Read the model definition and answer for the solid it produces. Units are mm, in the model's axes. A direction names the side the tool comes from. Coordinates: 2 decimals unless noted, no trailing zeros. Write each loop counter-clockwise with the first axis right and the second up, starting at its lowest first coordinate (ties: lowest second). Pieces come first, ordered by that corner, then holes.
(1) Given pin 1 (5.5 mm diameter, centred on y = 16.5, z = -23.5, fed in from +X); pin 2 (6 mm diameter, centred on x = 5.5, z = -14, fed in from +Y); pin 3 (2 mm diameter, centred on x = 3, y = 2.5, fed in from -Z); pin 4 (3.5 mm diameter, centred on x = -1.5, z = -19.5, fed in from -Y), each flat-ended and moving along its own axis, determine where each tip first touches the part or whether it passes through.
(2) Determine the mould class of faces 6 (the cylindrical face through (15.08, 0.09, -4.19)), 7 (the flat face through (-2, 20, -36.5)), 8 (the cylindrical face through (-1.522, 19.546, -32.085)) for opening direction Z: pulls with the +Z half, pulls with the -Z half, needs draft (parallel to the pull), parting line crosses it, or undercut.
(3) The part is cut by section B-B, the plane y = 0. Determine the outline of the cut face in (x, z), and give its area (3 significant figures).
(4) Which of the six approach directions +Z, -Z, +X, -X, +Y, -Y give full straight-line access (tool end or side, diameter ignored) to faces 1 (the flat face through (-10, 4.25, -4)), 2 (the flat face through (-1, 6, 0)), 3 (the flat face through (-2, 16.25, -22)), 4 (the flat face through (0, -4.25, -4)), 5 (the flat face through (4.032, 17, -13))?
(5) Straight lines are drawn through the part: line 1 along X through (y, z) = (20.5, -15); line 2 along X through (y, z) = (18.25, -33.5); line 3 along Z through (x, y) = (-1, 18.25). For each, find the intervals that lie inside material, in ascending order.
(6) The part is cut by section D-D, the plane z = -7. Determine the outline of the cut face in (x, y).
(7) The part is cut by section A-A, the plane z = -15. Determine the outline of the cut face in (x, y).
(8) The part is cut by section C-C, the plane x = -5. Determine the outline of the cut face in (y, z), and give its area (4 significant figures).
```python
from build123d import *

# Parameters (mm, degrees)
SKETCH_1_R          = 2.365979381
EXTRUDE_1_DEPTH     = 8.5
SKETCH_3_W          = 12
SKETCH_3_H          = 6.5
EXTRUDE_3_DEPTH     = 36.5
SKETCH_4_R          = 1.483814058
SKETCH_4_R_2        = 1.813860949
CUT_EXTRUDE_1_DEPTH = 49.146499311
FILLET_1_R          = 2


with BuildPart() as part:
    # 草圖1 → 填料-伸長1 (new body)
    with BuildSketch(Plane.XY):
        with BuildLine():
            Line((10.832162564, -4.25), (-11.776084859, -4.25))
            ThreePointArc((-11.776084859, -4.25), (-16.026084859, 0), (-11.776084859, 4.25))
            Line((-11.776084859, 4.25), (-7.967837436, 4.25))
            Line((-7.967837436, 4.25), (-7.967837436, 16.25))
            Line((-7.967837436, 16.25), (4.032162564, 16.25))
            Line((4.032162564, 16.25), (4.032162564, 4.25))
            Line((4.032162564, 4.25), (10.832162564, 4.25))
            ThreePointArc((10.832162564, 4.25), (15.082162564, 0), (10.832162564, -4.25))
        make_face()
        with Locations((10.832162564, 0)):
            Circle(SKETCH_1_R, mode=Mode.SUBTRACT)
    extrude(amount=-EXTRUDE_1_DEPTH)

    # 草圖3 → 填料-伸長3 (add)
    with BuildSketch(Plane.XY):
        with Locations((-1.967837436, 19.5)):
            Rectangle(SKETCH_3_W, SKETCH_3_H)
    extrude(amount=-EXTRUDE_3_DEPTH)

    # 草圖4 → 除料-伸長1 (cut, through all)
    with BuildSketch(Plane(origin=(0, 22.75, 0), x_dir=(1, 0, 0), z_dir=(0, 1, 0))):
        with Locations(Location((-1.967837436, 33.5, 0), (0, 0, 270))):
            Circle(SKETCH_4_R)
        with Locations(Location((-1.967837436, 15, 0), (0, 0, 270))):
            Circle(SKETCH_4_R_2)
    extrude(amount=-CUT_EXTRUDE_1_DEPTH, mode=Mode.SUBTRACT)

    # 圓角1
    fillet_1_edges = [part.edges().sort_by_distance(p)[0] for p in [
        (-7.967837436, 19.5, -36.5),
        (4.032162564, 19.5, -36.5),
    ]]
    fillet(fillet_1_edges, radius=FILLET_1_R)


solid = part.part
```
Computed:
1. pin 1: stops at x = 4.03
1. pin 2: stops at y = 22.75
1. pin 3: stops at z = -8.5
1. pin 4: stops at y = 16.25
2. face 6: needs draft
2. face 7: pulls with the -Z half
2. face 8: undercut
3. outline: (-16.03, -8.5) - (8.47, -8.5) - (8.47, 0) - (-16.03, 0) - close; (13.2, -8.5) - (15.08, -8.5) - (15.08, 0) - (13.2, 0) - close
3. area: 224 mm2
4. face 1: +Z, -Z, -X, +Y
4. face 2: +Z, +X, -X, +Y, -Y
4. face 3: -Z, +X, -X, -Y
4. face 4: +Z, -Z, +X, -X, -Y
4. face 5: +Z, -Z, +X, +Y
5. line 1: x = -7.97 to -3.78, -0.15 to 4.03
5. line 2: x = -7.97 to -3.45, -0.48 to 4.03
5. line 3: z = -36.5 to -34.62, -32.38 to -16.53, -13.47 to 0
6. outline: (-11.78, -4.25) - (10.83, -4.25) arc R4.25 ccw to (10.83, 4.25) - (4.03, 4.25) - (4.03, 22.75) - (-7.97, 22.75) - (-7.97, 4.25) - (-11.78, 4.25) arc R4.25 ccw to start; hole circle Ø4.73 at (10.83, 0)
7. outline: (-7.97, 16.25) - (-3.78, 16.25) - (-3.78, 22.75) - (-7.97, 22.75) - close; (-0.15, 16.25) - (4.03, 16.25) - (4.03, 22.75) - (-0.15, 22.75) - close
8. outline: (-4.25, -8.5) - (16.25, -8.5) - (16.25, -36.5) - (22.75, -36.5) - (22.75, 0) - (-4.25, 0) - close
8. area: 411.5 mm2
